```python
from build123d import *

# Parameters (mm, degrees)
F0_W     = 50.8
F0_H     = 25.4
F1_DEPTH = 76.2
F3_DEPTH = 76.2
F5_DEPTH = 25.4


with BuildPart() as f1:
    # F0 (on Front) → F1 (new body)
    with BuildSketch(Plane.XZ):
        Polygon((0, 50.8), (0, 0), (25.4, 0), (25.4, 25.4), (25.4, 50.8), align=None)
        Polygon((152.4, 50.8), (25.4, 50.8), (25.4, 25.4), (76.2, 25.4), (76.2, 0), (152.4, 0), align=None)
        with Locations((50.8, 12.7)):
            Rectangle(F0_W, F0_H)
    extrude(amount=-F1_DEPTH)

    # F2 (on face) → F3 (cut)
    with BuildSketch(Plane.XY.offset(50.8)):
        Polygon((152.4, 0), (152.4, 50.8), (76.2, 50.8), (25.4, 25.4), (25.4, 0), align=None)
    extrude(amount=-F3_DEPTH, mode=Mode.SUBTRACT)

    # F4 (on face) → F5 (cut)
    with BuildSketch(Plane.XY.offset(50.8)):
        Polygon((25.4, 50.8), (25.4, 25.4), (76.2, 50.8), align=None)
    extrude(amount=-F5_DEPTH, mode=Mode.SUBTRACT)


solid = f1.part
```
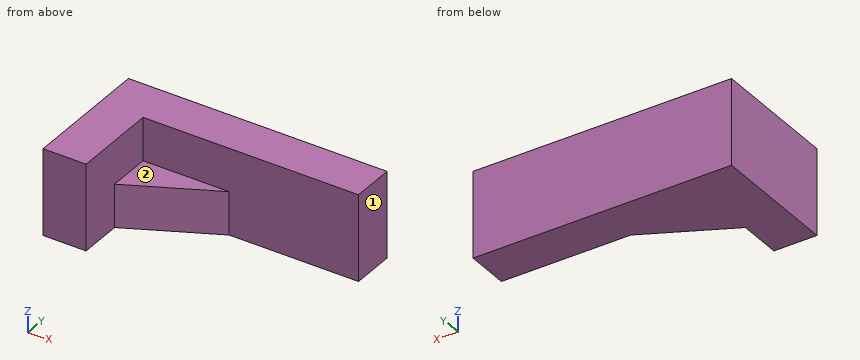
The listing builds one solid part. Answer for the finished solid, in the listing's coordinates (mm). Face numbers are marked on the shaded views. A direction names the side the tool comes from. Give positions to 0.01 mm unless a question says otherwise; leave off trailing zeros. Loops run counter-clockwise (first coordinate to the right, second up) from the corner with the lowest first, then second, coordinate; pieces in that order, holes last. Notation, with made-up numbers: M -33,84 L -11,84 A36 cw -11,119 Z; hole C 15.25,29 d11. An arc over 180 degrees is marked long. One line per item, written item: value.
1. Find the intervals of material crossed by probe 1 along Y at (x, z) = (140, 16.5); probe 2 along X at (y, z) = (48.5, 39); probe 3 along Y at (x, z) = (45.5, 13.5), in increasing order.
Found:
probe 1: 50.8 to 76.2
probe 2: 0 to 25.4
probe 3: 35.45 to 76.2
2. Section A-A on z = 13.5 is taken. Determine the outline of the cut face in (x, y).
Found:
outline: M 0,0 L 25.4,0 L 25.4,25.4 L 76.2,50.8 L 152.4,50.8 L 152.4,76.2 L 0,76.2 Z
3. Section D-D on x = 98 is taken. Determine the outline of the cut face in (y, z).
Found:
outline: M 50.8,0 L 76.2,0 L 76.2,50.8 L 50.8,50.8 Z
4. Section B-B on y = 36 is taken. Determine the outline of the cut face in (x, z).
Found:
outline: M 0,0 L 46.6,0 L 46.6,25.4 L 25.4,25.4 L 25.4,50.8 L 0,50.8 Z
5. For the marked faces 1 and 2, determine the directions among +Z, -Z, +X, -X, +Y, -Y from which every point of the face is accessible in a straight line to the end or side of a thin tool.
Found:
face 1: +Z, -Z, +X, +Y, -Y
face 2: +Z, +X, -Y
6. Each of these flat-tipped pins is pushed along its axis until it touches: P1, Ø3, axis at y = 38, z = 39, coming from the +X side; P2, Ø5, axis at y = 38, z = 15.5, coming from the +X side; P3, Ø10, axis at y = 31, z = 12, coming from the +X side. Where does it stop, or does it pass through?
Found:
P1: x = 25.4
P2: x = 55.6
P3: x = 46.6
7. Section C-C on x = 46.5 is taken. Determine the outline of the cut face in (y, z), plus the area to 3 significant figures.
Found:
outline: M 35.95,0 L 76.2,0 L 76.2,50.8 L 50.8,50.8 L 50.8,25.4 L 35.95,25.4 Z
area: 1,670 mm^2
